CAD build for the part. Positions are in the model's coordinates, mm. A direction names the side the tool comes from. Coordinates: 2 decimals unless noted, no trailing zeros. Loops run counter-clockwise (first coordinate to the right, second up) from the corner with the lowest first, then second, coordinate; pieces in that order, holes last. Notation, with made-up numbers: (70.5, 15.5) -> (114.5, 15.5) arc R38 cw to (114.5, 54.5) -> close; hole circle Ø2 at (-3, -1). An arc over 180 degrees is marked (long way). Answer as CSV lines item,"result". Start each with the question number.
```python
from build123d import *

# Parameters (mm, degrees)
F1_DEPTH = 25.4
F3_R     = 6.35
F2_R     = 6.35
F5_DEPTH = 25.4
F4_R     = 6.35
F6_DEPTH = 25.4


with BuildPart() as f1:
    # F0 (on Front) → F1 (new body)
    with BuildSketch(Plane.XZ):
        Polygon((0, 12.7), (0, 0), (76.2, 0), (76.2, 12.7), (50.8, 12.7), (50.8, 45.939504), (25.4, 45.939504), (25.4, 12.7), align=None)
    extrude(amount=F1_DEPTH)

    # F3 (on face) + F2 (on face) → F5 (cut)
    with BuildSketch(Plane.XY.offset(12.7)):
        with BuildLine():
            ThreePointArc((0, -12.7), (3.719744, -3.719744), (12.7, 0))
            Line((12.7, 0), (0, 0))
            Line((0, 0), (0, -12.7))
        make_face()
        with Locations((12.7, -12.7)):
            Circle(F3_R)
        with BuildLine():
            ThreePointArc((12.7, -25.4), (3.719744, -21.680256), (0, -12.7))
            Line((0, -12.7), (0, -25.4))
            Line((0, -25.4), (12.7, -25.4))
        make_face()
    with BuildSketch(Plane.XY.offset(12.7)):
        with Locations((63.5, -12.7)):
            Circle(F2_R)
        with BuildLine():
            ThreePointArc((63.5, 0), (72.480256, -3.719744), (76.2, -12.7))
            Line((76.2, -12.7), (76.2, 0))
            Line((76.2, 0), (63.5, 0))
        make_face()
        with BuildLine():
            ThreePointArc((76.2, -12.7), (72.480256, -21.680256), (63.5, -25.4))
            Line((63.5, -25.4), (76.2, -25.4))
            Line((76.2, -25.4), (76.2, -12.7))
        make_face()
    extrude(amount=-F5_DEPTH, mode=Mode.SUBTRACT)

    # F4 (on face) → F6 (cut)
    with BuildSketch(Plane.YZ.offset(50.8)):
        with Locations((-12.7, 31.75)):
            Circle(F4_R)
        with BuildLine():
            ThreePointArc((-12.7, 45.939504), (-3.719744, 42.21976), (0, 33.239504))
            Line((0, 33.239504), (0, 45.939504))
            Line((0, 45.939504), (-12.7, 45.939504))
        make_face()
        with BuildLine():
            ThreePointArc((-25.4, 33.239504), (-21.680256, 42.21976), (-12.7, 45.939504))
            Line((-12.7, 45.939504), (-25.4, 45.939504))
            Line((-25.4, 45.939504), (-25.4, 33.239504))
        make_face()
    extrude(amount=-F6_DEPTH, mode=Mode.SUBTRACT)


solid = f1.part
```
Q1. Two-plate mould, pull along X, no slides. Class faces 4 (the flat face through (25.4, -9.7, 25.9)), 5 (the cylindrical face through (62.12, -18.9, 6.44)), 6 (the flat face through (38, -25.4, 13)): pulls with the +X half, pulls with the -X half, needs draft (parallel to the pull), parting line crosses it, or undercut.
Q2. Saw through at C-C (z = 31.75). List the corners of the cut face in (x, y), and give its area (3 significant figures).
Q3. Probe probe 1 along X at (y, z) = (-7.25, 5); probe 2 along Y at (x, z) = (12.7, 8.5); probe 3 along Z at (x, y) = (43, -12.7). List the from-to ranges inside material, lowest first. Write a range as from..to.
Q4. Saw through at B-B (y = -15.75). List the corners of the cut face in (x, z).
Q5. Pin check, flat tips, straight feed: pin 1 Ø14.5 at (y, z) = (-12.7, 31.75) entering from +X; pin 2 Ø8 at (y, z) = (-13.5, 36.5) entering from -X. Stop position of each tip, or through.
Q6. Which spindle directions (+Z, -Z, +X, -X, +Y, -Y) get a long thin tool onto all of the face, cutting with end or side? Do faces 1 (the flat face through (55, -13, 12.7)), 2 (the flat face through (38, 0, 13)), 3 (the flat face through (19, -15, 12.7)). Say none if no direction does.
Q7. Saw through at D-D (x = 33). List the corners of the cut face in (y, z).
Q8. Saw through at A-A (z = 10.5). List the corners of the cut face in (x, y), and give its area (3 significant figures).
Ans:
1,face 4,"pulls with the -X half"
1,face 5,"undercut"
1,face 6,"needs draft"
2,outline,"(25.4, -25.4) -> (50.8, -25.4) -> (50.8, -19.05) -> (25.4, -19.05) -> close; (25.4, -6.35) -> (50.8, -6.35) -> (50.8, 0) -> (25.4, 0) -> close"
2,area,"323 mm²"
3,probe 1,"x = 1.23..9.44, 15.96..60.24, 66.76..74.97"
3,probe 2,"y = -25.4..-19.05, -6.35..0"
3,probe 3,"z = 0..25.4, 38.1..45.94"
4,outline,"(0.37, 0) -> (7.13, 0) -> (7.13, 12.7) -> (0.37, 12.7) -> close; (18.27, 0) -> (57.93, 0) -> (57.93, 12.7) -> (50.8, 12.7) -> (50.8, 26.18) -> (25.4, 26.18) -> (25.4, 12.7) -> (18.27, 12.7) -> close; (25.4, 37.32) -> (50.8, 37.32) -> (50.8, 45.57) -> (25.4, 45.57) -> close; (69.07, 0) -> (75.83, 0) -> (75.83, 12.7) -> (69.07, 12.7) -> close"
5,pin 1,"stops at x = 50.8"
5,pin 2,"stops at x = 25.4"
6,face 1,"+Z, +X, +Y, -Y"
6,face 2,"+Z, -Z, +X, -X, +Y"
6,face 3,"+Z, -X, +Y, -Y"
7,outline,"(-25.4, 0) -> (0, 0) -> (0, 33.24) arc R12.7 ccw to (-25.4, 33.24) -> close; hole circle Ø12.7 at (-12.7, 31.75)"
8,outline,"(12.7, -25.4) -> (63.5, -25.4) arc R12.7 ccw to (63.5, 0) -> (12.7, 0) arc R12.7 ccw to start; hole circle Ø12.7 at (12.7, -12.7); hole circle Ø12.7 at (63.5, -12.7)"
8,area,"1,540 mm²"
